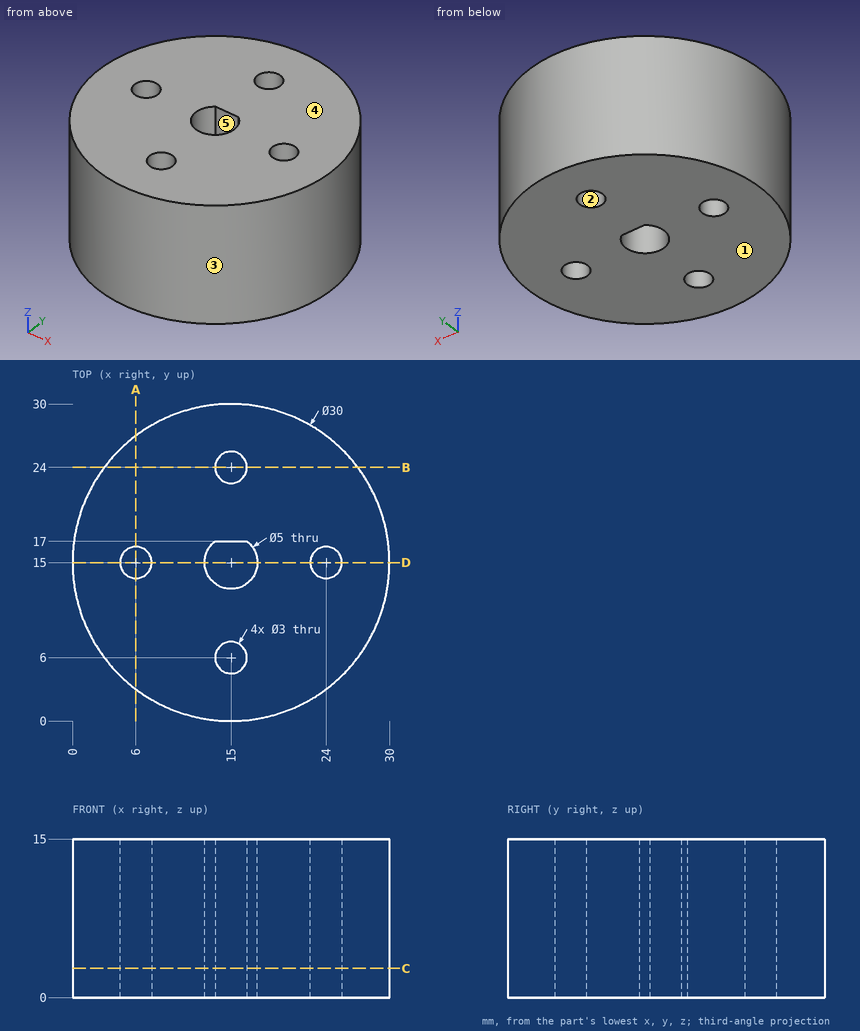
Answer from the drawing. Dimensions are ordinates in mm from the lowest x, y and z of the part. A direction names the side the tool comes from. Give positions to 0.01 mm unless a question says otherwise; leave off trailing zeros. Loops run counter-clockwise (first coordinate to the right, second up) from the corner with the lowest first, then second, coordinate; pieces in that order, holes last. Notation, with made-up numbers: (7, 21) -> (62, 21) arc R22 ccw to (62, 44) -> close; hole circle Ø9 at (40, 49). An arc over 180 degrees is marked (long way). Use a Markdown table: item, result.
Q1. Each of these flat-tipped pins is pushed along its axis until it touches: pin 1 (2.5 mm diameter, centred on x = 24, y = 15, fed in from +Z); pin 2 (4 mm diameter, centred on x = 11, z = 11.5, fed in from -Y); pin 3 (1.5 mm diameter, centred on x = 16, z = 7.5, fed in from +Y); pin 4 (3 mm diameter, centred on x = 12.5, z = 10.5, fed in from -Y). Where does it stop, or does it pass through?
Solved:
| item | result |
|---|---|
| pin 1 | passes through |
| pin 2 | stops at y = 0.13 |
| pin 3 | stops at y = 30 |
| pin 4 | stops at y = 0.03 |
Q2. Section D-D, the plane y = 15 is taken. Determine the outline of the cut face in (x, z).
Solved:
| item | result |
|---|---|
| outline | (0, 0) -> (4.5, 0) -> (4.5, 15) -> (0, 15) -> close; (7.5, 0) -> (12.5, 0) -> (12.5, 15) -> (7.5, 15) -> close; (17.5, 0) -> (22.5, 0) -> (22.5, 15) -> (17.5, 15) -> close; (25.5, 0) -> (30, 0) -> (30, 15) -> (25.5, 15) -> close |
Q3. Section C-C, the plane z = 2.75 is taken. Determine the outline of the cut face in (x, y), then the cut area to 3 significant figures.
Solved:
| item | result |
|---|---|
| outline | circle Ø30 at (15, 15); hole circle Ø3 at (6, 15); hole circle Ø3 at (15, 6); hole (13.5, 17) arc R2.5 ccw (long way) to (16.5, 17) -> close; hole circle Ø3 at (15, 24); hole circle Ø3 at (24, 15) |
| area | 660 mm^2 |
Q4. Determine the mould class of the marked faces 1, 2 and 3 for opening direction X: pulls with the +X half, pulls with the -X half, needs draft (parallel to the pull), parting line crosses it, or undercut.
Solved:
| item | result |
|---|---|
| face 1 | needs draft |
| face 2 | undercut |
| face 3 | parting line crosses it |
Q5. Section A-A, the plane x = 6 is taken. Determine the outline of the cut face in (y, z), then the cut area to 3 significant figures.
Solved:
| item | result |
|---|---|
| outline | (3, 0) -> (13.5, 0) -> (13.5, 15) -> (3, 15) -> close; (16.5, 0) -> (27, 0) -> (27, 15) -> (16.5, 15) -> close |
| area | 315 mm^2 |
Q6. A tool of negligible diameter and unlimited length cuts with its end or side. For the marked faces 4 and 5, from which of +Z, -Z, +X, -X, +Y, -Y can it reach the whole face along a straight path? Write none if from no direction.
Solved:
| item | result |
|---|---|
| face 4 | +Z, +X, -X, +Y, -Y |
| face 5 | +Z, -Z |
Q7. Find the intervals of material crossed by line 1 along Y through (x, z) = (14.25, 6.25); line 2 along Y through (x, z) = (15, 3.5); line 3 along X through (y, z) = (24.5, 13), in increasing order.
Solved:
| item | result |
|---|---|
| line 1 | y = 0.02 to 4.7, 7.3 to 12.62, 17 to 22.7, 25.3 to 29.98 |
| line 2 | y = 0 to 4.5, 7.5 to 12.5, 17 to 22.5, 25.5 to 30 |
| line 3 | x = 3.39 to 13.59, 16.41 to 26.61 |
